For this review, take the finished solid that the model builds, in its own axes (mm). Face numbers are marked on the shaded views. A direction names the side the tool comes from. Round coordinates to 2 decimals unless told otherwise and drop trailing zeros. Order: outer loops, then holes, each group sorted by start corner. A loop starts at its lowest first (then second) coordinate and runs counter-clockwise, first axis right, second up. Notation, with made-up numbers: (-38.5, -5) -> (-6.5, -5) arc R33 cw to (-6.5, 23) -> close; hole circle Ø9 at (29, -22.75). An arc over 180 degrees is marked (long way). Use a Markdown table: item, result. Add a question column.
1) Machinability: for the marked faces 1, 2 and 3, which of the approach directions +Z, -Z, +X, -X, +Y, -Y give a long, thin tool a straight path to every point of the face, cutting with its end or side? Answer none if there is none.
2) Consider section D-D (z = -50.5). State the section outline as (x, y) points, plus the area to 3 significant figures.
3) Draft analysis for pull direction X (two halves, no side actions). For the marked faces 4, 5 and 6, state which applies: pulls with the +X half, pulls with the -X half, needs draft (parallel to the pull), parting line crosses it, or undercut.
4) Clearance check with flat-ended pins moving along their axes: P1, Ø7, axis at x = 40, z = -5, coming from the +Y side; P2, Ø0.9, axis at x = 76.5, z = -45.5, coming from the +Y side; P3, Ø5, axis at x = 59, y = 20.5, coming from the -Z side. State where each tip first meets the part, or that it passes through.
5) Wall thickness on line 1 along X through (y, z) = (7, -10); line 2 along X through (y, z) = (7.75, -15); line 3 along X through (y, z) = (27, -22.5): over which ranges is each line inside the solid? List them lowest first. Write a range as [from, to].
6) Consider section C-C (x = 6). State the section outline as (y, z) points, plus the area to 3 significant figures.
7) Consider section A-A (z = -5). State the section outline as (x, y) points.
8) Consider section B-B (x = 40). State the section outline as (y, z) points.
```python
from build123d import *

# Parameters (mm, degrees)
SKETCH1_W           = 80
SKETCH1_H           = 60
BOSS_EXTRUDE1_DEPTH = 10
BOSS_EXTRUDE2_DEPTH = 10
LPATTERN1_COUNT     = 2
LPATTERN1_PITCH     = 70
BOSS_EXTRUDE3_START = -30
BOSS_EXTRUDE3_DEPTH = 5
FILLET1_R           = 10
SKETCH4_R           = 2.739205113
CUT_EXTRUDE1_DEPTH  = 11
CUT_EXTRUDE2_DEPTH  = 81


with BuildPart() as part:
    # Sketch1 → Boss-Extrude1 (new body)
    with BuildSketch(Plane(origin=(0, 0, 0), x_dir=(1, 0, 0), z_dir=(0, 1, 0))):
        with Locations((40, 30)):
            Rectangle(SKETCH1_W, SKETCH1_H)
    extrude(amount=BOSS_EXTRUDE1_DEPTH)

    # Sketch2 → Boss-Extrude2 (add)
    with BuildSketch(Plane(origin=(0, 0, 0), x_dir=(0, 0, -1), z_dir=(1, 0, 0))):
        Polygon((0, 10), (30, 40), (60, 10), align=None)
    boss_extrude2 = extrude(amount=BOSS_EXTRUDE2_DEPTH)

    # LPattern1: Boss-Extrude2 ×2
    with Locations(*[(i * LPATTERN1_PITCH, 0, 0) for i in range(1, LPATTERN1_COUNT)]):
        add(boss_extrude2)

    # Sketch3 → Boss-Extrude3 (add, symmetric)
    with BuildSketch(Plane.XY.offset(BOSS_EXTRUDE3_START)):
        with BuildLine():
            Line((10, 30), (10, 10))
            Line((10, 10), (70, 10))
            Line((70, 10), (70, 30))
            ThreePointArc((70, 30), (40, 16.457513111), (10, 30))
        make_face()
    extrude(amount=BOSS_EXTRUDE3_DEPTH, both=True)

    # Fillet1
    fillet1_edges = [part.edges().sort_by_distance(p)[0] for p in [
        (5, 40, -30),
        (75, 40, -30),
    ]]
    fillet(fillet1_edges, radius=FILLET1_R)

    # Sketch4 → Cut-Extrude1 (cut, through all)
    with BuildSketch(Plane(origin=(0, 10, 0), x_dir=(1, 0, 0), z_dir=(0, 1, 0))):
        with Locations((40, 15)):
            Circle(SKETCH4_R)
        with Locations((45, 10)):
            Circle(SKETCH4_R)
        with Locations((40, 5)):
            Circle(SKETCH4_R)
        with Locations((35, 10)):
            Circle(SKETCH4_R)
    extrude(amount=-CUT_EXTRUDE1_DEPTH, mode=Mode.SUBTRACT)

    # Sketch5 → Cut-Extrude2 (cut, through all)
    with BuildSketch(Plane(origin=(0, 0, 0), x_dir=(0, 0, -1), z_dir=(1, 0, 0))):
        Polygon((46.5, 12.401923789), (48, 15), (46.5, 17.598076211), (43.5, 17.598076211), (42, 15), (43.5, 12.401923789), align=None)
    extrude(amount=CUT_EXTRUDE2_DEPTH, mode=Mode.SUBTRACT)


solid = part.part
```
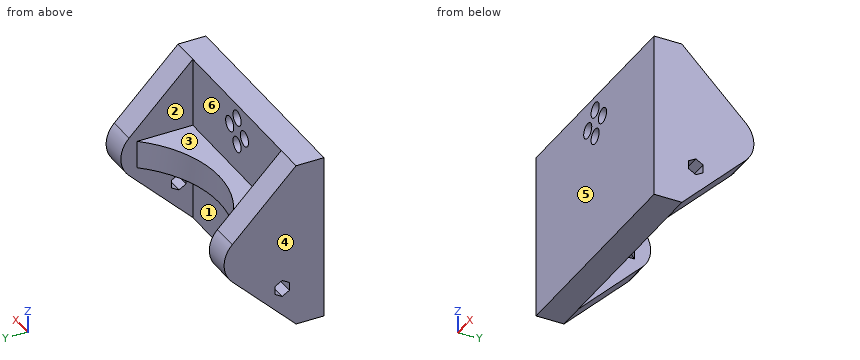
Results list:
| question | item | result |
|---|---|---|
| 1 | face 1 | -Z, +Y |
| 1 | face 2 | +Y |
| 1 | face 3 | +Z, +Y |
| 2 | outline | (0, 0) -> (80, 0) -> (80, 19.5) -> (70, 19.5) -> (70, 10) -> (10, 10) -> (10, 19.5) -> (0, 19.5) -> close |
| 2 | area | 990 mm2 |
| 3 | face 4 | pulls with the -X half |
| 3 | face 5 | needs draft |
| 3 | face 6 | undercut |
| 4 | P1 | y = 10 |
| 4 | P2 | y = 24.95 |
| 4 | P3 | z = -35 |
| 5 | line 1 | [0, 32.26], [37.74, 42.26], [47.74, 80] |
| 5 | line 2 | [0, 37.26], [42.74, 80] |
| 5 | line 3 | [0, 10], [70, 80] |
| 6 | outline | (0, -60) -> (10, -60) -> (32.93, -37.07) arc R10 ccw to (32.93, -22.93) -> (10, 0) -> (0, 0) -> close; hole (12.4, -46.5) -> (15, -48) -> (17.6, -46.5) -> (17.6, -43.5) -> (15, -42) -> (12.4, -43.5) -> close |
| 6 | area | 1,460 mm2 |
| 7 | outline | (0, 0) -> (37.26, 0) -> (37.26, 10) -> (10, 10) -> (10, 15) -> (0, 15) -> close; (42.74, 0) -> (80, 0) -> (80, 15) -> (70, 15) -> (70, 10) -> (42.74, 10) -> close |
| 8 | outline | (0, -60) -> (10, -60) -> (10, -35) -> (16.46, -35) -> (16.46, -25) -> (10, -25) -> (10, -17.74) -> (0, -17.74) -> close; (0, -12.26) -> (10, -12.26) -> (10, -7.74) -> (0, -7.74) -> close; (0, -2.26) -> (10, -2.26) -> (10, 0) -> (0, 0) -> close |
